For this review, take the finished solid that the model builds, in its own axes (mm). Give positions to 0.01 mm unless a question says otherwise; leave off trailing zeros. Use CSV: the item, a comma, the result in double quotes. Start each with the question number.
1. Insertion check: P1, Ø3.5, axis at x = 0, y = -10, coming from the +Z side; P2, Ø3, axis at x = 1, z = -309.5, coming from the +Y side; P3, Ø1.8, axis at x = 0.5, z = -359.5, coming from the -Y side. Each pin has a flat end and moves straight along its axis. Give the tip position at first contact, or say it passes through.
2. To check wall thickness, follow line 1 (Y direction, x = -8.25, z = -190.5); line 2 (Y direction, x = 0, z = -323); line 3 (Y direction, x = 7.5, z = -180.5). State the ranges of each line that lie inside material, in increasing order. Write a range as [from, to].
3. Take a section at A-A, the plane z = -143.5. State how many separate pieces and enclosed holes the cut face has, and give its area (3 significant figures).
4. The part is to be moulded in two halves that separate along Z. For faces 1 (the face through (-5, 5, 0)), 2 (the face through (-10, 0, -246)), 3 (the face through (-5, 5, -500)), say which applies: pulls with the +Z half, pulls with the -Z half, needs draft (parallel to the pull), parting line crosses it, or undercut.
Autodesk Inventor part; units mm, degrees
ref_plane "C1_XY" through (0, 0, 0) normal (0, 0, 1) x (1, 0, 0)
ref_plane "C1_YZ" through (0, 0, 0) normal (1, 0, 0) x (0, 1, 0)
ref_plane "C1_ZX" through (0, 0, 0) normal (0, 1, 0) x (0, 0, 1)
sketch "Sketch_1" plane through (0, 0, 0) normal (0, 0, 1) x (1, 0, 0)
  line L0 (-10, -7) -> (-8, -7)
  line L1 (-8, -7) -> (-8, -4)
  line L2 (-8, -4) -> (-7.0607, -4)
  line L3 (-7.0607, -4) -> (-4, -7.0607)
  line L4 (-4, -7.0607) -> (-4, -9.4804)
  line L5 (-4, -9.4804) -> (-3.7, -10)
  line L6 (-3.7, -10) -> (-4, -10.5196)
  line L7 (-4, -10.5196) -> (-4, -12.9393)
  line L8 (-4, -12.9393) -> (-7.0607, -16)
  line L9 (-7.0607, -16) -> (-8, -16)
  line L10 (-8, -16) -> (-8, -13)
  line L11 (-8, -13) -> (-10, -13)
  line L12 (-10, -13) -> (-10, -19)
  arc A0 (-10, -19) -> (-9, -20) centre (-9, -19) ccw
  line L13 (-9, -20) -> (-3, -20)
  line L14 (-3, -20) -> (-3, -18)
  line L15 (-3, -18) -> (-6, -18)
  line L16 (-6, -18) -> (-6, -17.0607)
  line L17 (-6, -17.0607) -> (-2.9393, -14)
  line L18 (-2.9393, -14) -> (-0.5196, -14)
  line L19 (-0.5196, -14) -> (0, -13.7)
  line L20 (0, -13.7) -> (0.5196, -14)
  line L21 (0.5196, -14) -> (2.9393, -14)
  line L22 (2.9393, -14) -> (6, -17.0607)
  line L23 (6, -17.0607) -> (6, -18)
  line L24 (6, -18) -> (3, -18)
  line L25 (3, -18) -> (3, -20)
  line L26 (3, -20) -> (9, -20)
  arc A1 (9, -20) -> (10, -19) centre (9, -19) ccw
  line L27 (10, -19) -> (10, -13)
  line L28 (10, -13) -> (8, -13)
  line L29 (8, -13) -> (8, -16)
  line L30 (8, -16) -> (7.0607, -16)
  line L31 (7.0607, -16) -> (4, -12.9393)
  line L32 (4, -12.9393) -> (4, -10.5196)
  line L33 (4, -10.5196) -> (3.7, -10)
  line L34 (3.7, -10) -> (4, -9.4804)
  line L35 (4, -9.4804) -> (4, -7.0607)
  line L36 (4, -7.0607) -> (7.0607, -4)
  line L37 (7.0607, -4) -> (8, -4)
  line L38 (8, -4) -> (8, -7)
  line L39 (8, -7) -> (10, -7)
  line L40 (10, -7) -> (10, 7)
  line L41 (10, 7) -> (8, 7)
  line L42 (8, 7) -> (8, 4)
  line L43 (8, 4) -> (7.0607, 4)
  line L44 (7.0607, 4) -> (4, 7.0607)
  line L45 (4, 7.0607) -> (4, 9.4804)
  line L46 (4, 9.4804) -> (3.7, 10)
  line L47 (3.7, 10) -> (4, 10.5196)
  line L48 (4, 10.5196) -> (4, 12.9393)
  line L49 (4, 12.9393) -> (7.0607, 16)
  line L50 (7.0607, 16) -> (8, 16)
  line L51 (8, 16) -> (8, 13)
  line L52 (8, 13) -> (10, 13)
  line L53 (10, 13) -> (10, 19)
  arc A2 (10, 19) -> (9, 20) centre (9, 19) ccw
  line L54 (9, 20) -> (3, 20)
  line L55 (3, 20) -> (3, 18)
  line L56 (3, 18) -> (6, 18)
  line L57 (6, 18) -> (6, 17.0607)
  line L58 (6, 17.0607) -> (2.9393, 14)
  line L59 (2.9393, 14) -> (0.5196, 14)
  line L60 (0.5196, 14) -> (0, 13.7)
  line L61 (0, 13.7) -> (-0.5196, 14)
  line L62 (-0.5196, 14) -> (-2.9393, 14)
  line L63 (-2.9393, 14) -> (-6, 17.0607)
  line L64 (-6, 17.0607) -> (-6, 18)
  line L65 (-6, 18) -> (-3, 18)
  line L66 (-3, 18) -> (-3, 20)
  line L67 (-3, 20) -> (-9, 20)
  arc A3 (-9, 20) -> (-10, 19) centre (-9, 19) ccw
  line L68 (-10, 19) -> (-10, 13)
  line L69 (-10, 13) -> (-8, 13)
  line L70 (-8, 13) -> (-8, 16)
  line L71 (-8, 16) -> (-7.0607, 16)
  line L72 (-7.0607, 16) -> (-4, 12.9393)
  line L73 (-4, 12.9393) -> (-4, 10.5196)
  line L74 (-4, 10.5196) -> (-3.7, 10)
  line L75 (-3.7, 10) -> (-4, 9.4804)
  line L76 (-4, 9.4804) -> (-4, 7.0607)
  line L77 (-4, 7.0607) -> (-7.0607, 4)
  line L78 (-7.0607, 4) -> (-8, 4)
  line L79 (-8, 4) -> (-8, 7)
  line L80 (-8, 7) -> (-10, 7)
  line L81 (-10, 7) -> (-10, -7)
  line L82 (-8, 1.7) -> (-8, -1.7)
  arc A4 (-8, -1.7) -> (-7.7, -2) centre (-7.7, -1.7) ccw
  line L83 (-7.7, -2) -> (-7.0636, -2)
  arc A5 (-6.8515, -2.0879) -> (-7.0636, -2) centre (-7.0636, -2.3) ccw
  line L84 (-6.8515, -2.0879) -> (-2.9393, -6)
  line L85 (-2.9393, -6) -> (2.9393, -6)
  line L86 (2.9393, -6) -> (6.8515, -2.0879)
  arc A6 (7.0636, -2) -> (6.8515, -2.0879) centre (7.0636, -2.3) ccw
  line L87 (7.0636, -2) -> (7.7, -2)
  arc A7 (7.7, -2) -> (8, -1.7) centre (7.7, -1.7) ccw
  line L88 (8, -1.7) -> (8, 1.7)
  arc A8 (8, 1.7) -> (7.7, 2) centre (7.7, 1.7) ccw
  line L89 (7.7, 2) -> (7.0636, 2)
  arc A9 (6.8515, 2.0879) -> (7.0636, 2) centre (7.0636, 2.3) ccw
  line L90 (6.8515, 2.0879) -> (2.9393, 6)
  line L91 (2.9393, 6) -> (-2.9393, 6)
  line L92 (-2.9393, 6) -> (-6.8515, 2.0879)
  arc A10 (-7.0636, 2) -> (-6.8515, 2.0879) centre (-7.0636, 2.3) ccw
  line L93 (-7.0636, 2) -> (-7.7, 2)
  arc A11 (-7.7, 2) -> (-8, 1.7) centre (-7.7, 1.7) ccw
extrude "Extrusion1" add sketch "Sketch_1" against normal blind 500
sketch "Sketch2" plane through (0, 0, -500) normal (0, 0, -1) x (-1, 0, 0)
  point P0 (0, 10)
hole "Hole1" at (0, 10, -500) direction (0, 0, 1) diameter 4.2 depth 500
pattern_linear "Rectangular Pattern1" count 2 spacing 20 along (0, -1, 0) of "Hole1"
ref_plane "C1_XY" through (0, 0, 0) normal (0, 0, 1) x (1, 0, 0)
ref_plane "C1_YZ" through (0, 0, 0) normal (1, 0, 0) x (0, 1, 0)
ref_plane "C1_ZX" through (0, 0, 0) normal (0, 1, 0) x (0, 0, 1)
properties part number "HFS5-2040-500"
Result set:
1,P1,"through"
1,P2,"y = 14"
1,P3,"y = -14"
2,line 1,"[-20, -13], [-7, 7], [13, 20]"
2,line 2,"[-13.7, -12.1], [-7.9, -6], [6, 7.9], [12.1, 13.7]"
2,line 3,"[-20, -16], [-4, -2], [2, 4], [16, 20]"
3,separate pieces,"1"
3,enclosed holes,"3"
3,area,"324 mm2"
4,face 1,"pulls with the +Z half"
4,face 2,"needs draft"
4,face 3,"pulls with the -Z half"
